```python
from build123d import *

# Parameters (mm, degrees)
EXTRUDE1_DEPTH = 20
SHELL1_START   = 2.5
SHELL1_DEPTH   = 17.5
SKETCH2_R      = 2.5
EXTRUDE2_DEPTH = 225.675435256


# Read off the part's stored shape, not the designer's step: Shell1
with BuildPart() as part:
    # Sketch1 → Extrude1 (new body)
    with BuildSketch(Plane.XY):
        with BuildLine():
            Line((0, 0), (0, -85))
            ThreePointArc((0, -85), (1.464466094, -88.535533906), (5, -90))
            Line((5, -90), (148.660254038, -90))
            ThreePointArc((148.660254038, -90), (149.954349263, -90.170370869), (151.160254038, -90.669872981))
            Line((151.160254038, -90.669872981), (189.551270189, -112.834936491))
            ThreePointArc((189.551270189, -112.834936491), (192.051270189, -112.834936491), (193.301270189, -110.669872981))
            Line((193.301270189, -110.669872981), (193.301270189, -97.886751346))
            ThreePointArc((193.301270189, -97.886751346), (192.631397208, -95.386751346), (190.801270189, -93.556624327))
            Line((190.801270189, -93.556624327), (116.519237886, -50.669872981))
            ThreePointArc((116.519237886, -50.669872981), (115.313333112, -50.170370869), (114.019237886, -50))
            Line((114.019237886, -50), (55, -50))
            ThreePointArc((55, -50), (51.464466094, -48.535533906), (50, -45))
            Line((50, -45), (50, 0))
            Line((50, 0), (0, 0))
        make_face()
    extrude(amount=EXTRUDE1_DEPTH)

    # Shell1 outline → Shell1 (cut)
    with BuildSketch(Plane.XY.offset(SHELL1_START)):
        with BuildLine():
            Line((2.5, -2.5), (2.5, -85))
            ThreePointArc((2.5, -85), (3.232233047, -86.767766953), (5, -87.5))
            Line((5, -87.5), (148.660254038, -87.5))
            ThreePointArc((148.660254038, -87.5), (150.601396876, -87.755556303), (152.410254038, -88.504809472))
            Line((152.410254038, -88.504809472), (190.801270189, -110.669872981))
            Line((190.801270189, -110.669872981), (190.801270189, -97.886751346))
            ThreePointArc((190.801270189, -97.886751346), (190.466333699, -96.636751346), (189.551270189, -95.721687836))
            Line((189.551270189, -95.721687836), (115.269237886, -52.834936491))
            ThreePointArc((115.269237886, -52.834936491), (114.666285499, -52.585185434), (114.019237886, -52.5))
            Line((114.019237886, -52.5), (55, -52.5))
            ThreePointArc((55, -52.5), (49.696699141, -50.303300859), (47.5, -45))
            Line((47.5, -45), (47.5, -2.5))
            Line((47.5, -2.5), (2.5, -2.5))
        make_face()
    extrude(amount=SHELL1_DEPTH, mode=Mode.SUBTRACT)

    # Sketch2 → Extrude2 (cut, through all)
    with BuildSketch(Plane.XY.offset(2.5)):
        with Locations((15, -10)):
            Circle(SKETCH2_R)
        with Locations((35, -10)):
            Circle(SKETCH2_R)
    extrude(amount=-EXTRUDE2_DEPTH, mode=Mode.SUBTRACT)


solid = part.part
```
Build history of the part. All positions in model axes, mm. A direction names the side the tool comes from. Coordinates: 2 decimals unless noted, no trailing zeros. Write each loop counter-clockwise with the first axis right and the second up, starting at its lowest first coordinate (ties: lowest second). Pieces come first, ordered by that corner, then holes.
1. Drill centre lines: probe 1 along Y at (x, z) = (89, 18.25); probe 2 along X at (y, z) = (-8, 7.5); probe 3 along Y at (x, z) = (19, 7.5). Where is each one in solid material? Low to high.
Answer block:
probe 1: y = -90 to -87.5, -52.5 to -50
probe 2: x = 0 to 2.5, 47.5 to 50
probe 3: y = -90 to -87.5, -2.5 to 0
2. 3-axis set-ups, long thin cutter, end or side, ignore diameter. For faces 1 (the cylindrical face through (37.31, -10.96, 1.27)), 2 (the flat face through (85, -50, 10)), 3 (the flat face through (47.5, -24, 11)): which of +Z, -Z, +X, -X, +Y, -Y reach the whole face in a straight line?
Answer block:
face 1: +Z, -Z
face 2: +Z, -Z, +X, +Y
face 3: +Z
3. Band-saw the part on B-B, the plane y = -10. Give the cut face in (x, z).
Answer block:
outline: (0, 0) - (12.5, 0) - (12.5, 2.5) - (2.5, 2.5) - (2.5, 20) - (0, 20) - close; (17.5, 0) - (32.5, 0) - (32.5, 2.5) - (17.5, 2.5) - close; (37.5, 0) - (50, 0) - (50, 20) - (47.5, 20) - (47.5, 2.5) - (37.5, 2.5) - close
4. Band-saw the part on A-A, the plane x = 15. Give the cut face in (y, z).
Answer block:
outline: (-90, 0) - (-12.5, 0) - (-12.5, 2.5) - (-87.5, 2.5) - (-87.5, 20) - (-90, 20) - close; (-7.5, 0) - (0, 0) - (0, 20) - (-2.5, 20) - (-2.5, 2.5) - (-7.5, 2.5) - close
5. Drop flat-ended pins along their axis: pin 1 (5 mm diameter, centred on x = 84.5, z = 12.5, fed in from +Y); pin 2 (10 mm diameter, centred on x = 107, y = -42, fed in from +Z); pin 3 (8 mm diameter, centred on x = 35, y = -10, fed in from +Z); pin 4 (1.5 mm diameter, centred on y = -57.5, z = 3, fed in from +X). Give the stop position or say it passes through.
Answer block:
pin 1: stops at y = -50
pin 2: passes through
pin 3: stops at z = 2.5
pin 4: stops at x = 129.65
6. Pull direction X, two halves, no side cores. Call faces 4 (the flat face through (2.5, -43, 11)), 5 (the flat face through (76, -90, 10)), 6 (the cylindrical face through (52, -49, 10)): released by +X, released by -X, zero draft, split by the parting line, or undercut.
Answer block:
face 4: undercut
face 5: zero draft
face 6: released by +X
7. Band-saw the part on D-D, the plane x = 73.5. Give the cut face in (y, z), and give its area (4 significant figures).
Answer block:
outline: (-90, 0) - (-50, 0) - (-50, 20) - (-52.5, 20) - (-52.5, 2.5) - (-87.5, 2.5) - (-87.5, 20) - (-90, 20) - close
area: 187.5 mm2
8. Band-saw the part on C-C, the plane z = 14. Give the cut face in (x, y), and give its area (3 significant figures).
Answer block:
outline: (0, -85) arc R5 ccw to (5, -90) - (148.66, -90) arc R5 cw to (151.16, -90.67) - (189.55, -112.83) arc R2.5 ccw to (193.3, -110.67) - (193.3, -97.89) arc R5 ccw to (190.8, -93.56) - (116.52, -50.67) arc R5 ccw to (114.02, -50) - (55, -50) arc R5 cw to (50, -45) - (50, 0) - (0, 0) - close; hole (2.5, -85) arc R2.5 ccw to (5, -87.5) - (148.66, -87.5) arc R7.5 cw to (152.41, -88.5) - (190.8, -110.67) - (190.8, -97.89) arc R2.5 ccw to (189.55, -95.72) - (115.27, -52.83) arc R2.5 ccw to (114.02, -52.5) - (55, -52.5) arc R7.5 cw to (47.5, -45) - (47.5, -2.5) - (2.5, -2.5) - close
area: 1,370 mm2
